from build123d import *

# Parameters (mm, degrees)
SKETCH1_R                = 12.5
BOSS_EXTRUDE1_DEPTH      = 68
SKETCH2_R                = 12.5
BOSS_EXTRUDE2_DEPTH      = 34
BOSS_EXTRUDE2_DEPTH_BACK = 34


with BuildPart() as part:
    # Sketch1 → Boss-Extrude1 (new body)
    with BuildSketch(Plane.XY):
        Circle(SKETCH1_R)
    extrude(amount=BOSS_EXTRUDE1_DEPTH)

    # Sketch2 → Boss-Extrude2 (add, two sides)
    with BuildSketch(Plane(origin=(0, 0, 0), x_dir=(0, 0, -1), z_dir=(1, 0, 0))) as boss_extrude2_sk:
        with Locations((-34, 0)):
            Circle(SKETCH2_R)
    extrude(amount=BOSS_EXTRUDE2_DEPTH)
    extrude(boss_extrude2_sk.sketch, amount=-BOSS_EXTRUDE2_DEPTH_BACK)


solid = part.part
Design review of the part built by this model. Coordinates are the model's own, in mm. A direction names the side the tool comes from. Round coordinates to 2 decimals unless told otherwise and drop trailing zeros. Write each loop counter-clockwise with the first axis right and the second up, starting at its lowest first coordinate (ties: lowest second). Pieces come first, ordered by that corner, then holes. Notation, with made-up numbers: M 31.25,9 L 82.25,9 A22 cw 82.25,17 Z; hole C -26,-6.5 d8. An arc over 180 degrees is marked long. One line per item, written item: value. Start each with the question number.
1. Take a section at B-B on z = 37. State the section outline as (x, y) points.
2. Take a section at C-C on x = -10. State the section outline as (y, z) points, then the cut area to 3 significant figures.
3. To check wall thickness, follow probe 1 along Z at (x, y) = (13.5, 0.25); probe 2 along X at (y, z) = (3.75, 18); probe 3 along Z at (x, y) = (-12, 6). State the ranges of each line that lie inside material, in increasing order. Write a range as from..to.
4. Clearance check with flat-ended pins moving along their axes: P1, Ø5, axis at x = -26, y = 1.5, coming from the +Z side; P2, Ø4, axis at x = 7.5, z = 50, coming from the -Y side (3 decimals); P3, Ø8, axis at y = -2, z = 53.5, coming from the +X side. State where each tip first meets the part, or that it passes through.
5. Take a section at A-A on y = 0. State the section outline as (x, z) points.
6. For faces 1 (the face through (-1.627, 12.394, 12.984)), 2 (the face through (20.54, 12.394, 35.627)), 3 (the face through (-1.627, 12.394, 54.54)), list the 3-axis set-ups (+Z, -Z, +X, -X, +Y, -Y) from which the entire face can be reached by the end or side of a thin tool; tool diameter is ignored.
7. Take a section at D-D on y = -11. State the section outline as (x, z) points.
Computed:
1. outline: M -34,-12.13 L -3,-12.13 A12.5 ccw 3,-12.13 L 34,-12.13 L 34,12.13 L 3,12.13 A12.5 ccw -3,12.13 L -34,12.13 Z
2. outline: M -7.5,0 L 7.5,0 L 7.5,24 A12.5 ccw 7.5,44 L 7.5,68 L -7.5,68 L -7.5,44 A12.5 ccw -7.5,24 Z
2. area: 1,160 mm²
3. probe 1: z = 21.5..46.5
3. probe 2: x = -11.92..11.92
3. probe 3: z = 23.03..44.97
4. P1: stops at z = 46.5
4. P2: stops at y = -11.225
4. P3: stops at x = 12.5
5. outline: M -34,21.5 L -12.5,21.5 L -12.5,0 L 12.5,0 L 12.5,21.5 L 34,21.5 L 34,46.5 L 12.5,46.5 L 12.5,68 L -12.5,68 L -12.5,46.5 L -34,46.5 Z
6. face 1: -Z
6. face 2: +X
6. face 3: +Z
7. outline: M -34,28.06 L -5.94,28.06 L -5.94,0 L 5.94,0 L 5.94,28.06 L 34,28.06 L 34,39.94 L 5.94,39.94 L 5.94,68 L -5.94,68 L -5.94,39.94 L -34,39.94 Z
